The figure shows three views and two pictorial views of one solid part (mm, origin at its lowest corner). Answer the questions. A direction names the side the tool comes from. Give positions to 0.01 mm unless a question says otherwise; leave off trailing zeros. Write each loop counter-clockwise with the first axis right and the second up, starting at its lowest first coordinate (ties: lowest second). Pieces come first, ordered by that corner, then holes. Notation, with made-up numbers: (-16, 12.5) - (16, 12.5) arc R29 cw to (16, 35.5) - close; hole circle Ø5 at (-2, 79). An arc over 180 degrees is marked (long way). Use CSV: the item, a comma, the result in double quotes. Start each with the question number.
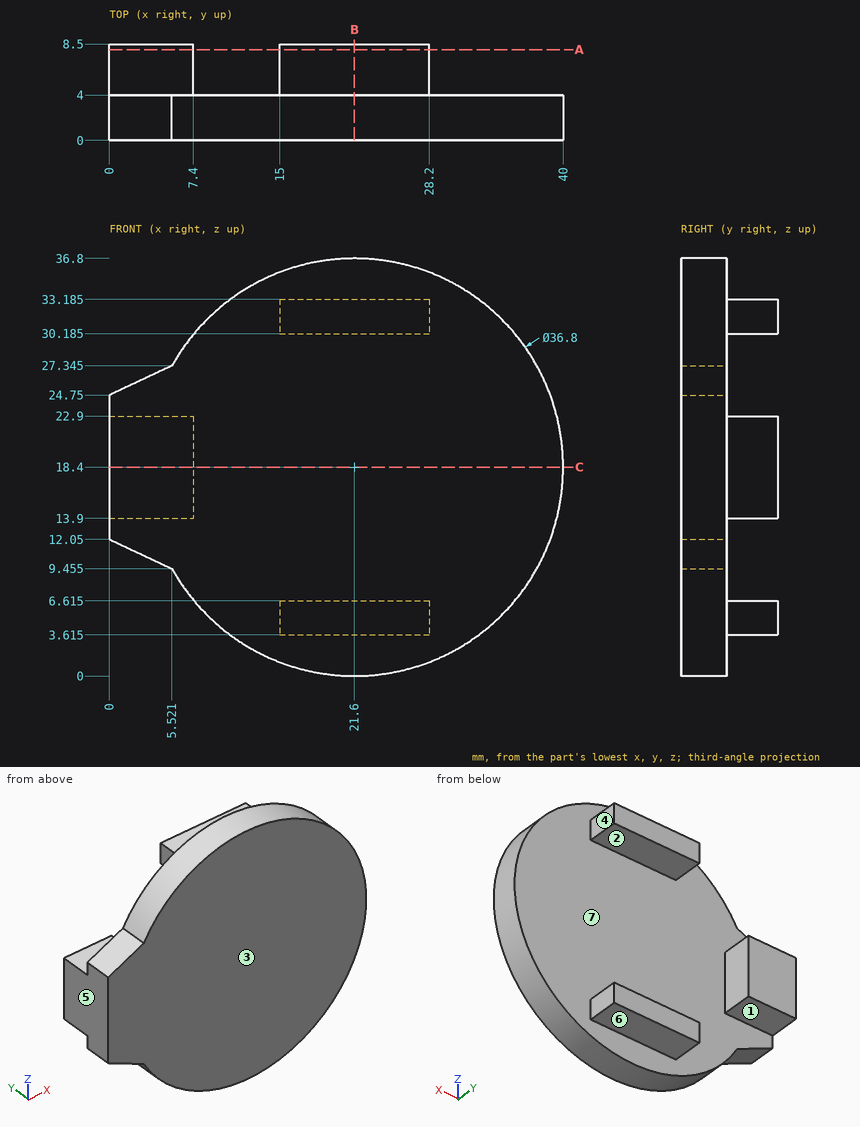
(1) Which of the six approach directions +Z, -Z, +X, -X, +Y, -Y give full straight-line access (tool end or side, diameter ignored) to the marked faces 1, 2, 3 and 4?
(2) For a pull along Z with two mould halves and no side action, classify the marked faces 5, 6 and 7 as pulls with the +Z half, pulls with the -Z half, needs draft (parallel to the pull), parting line crosses it, or undercut.
(3) The part is cut by section A-A on y = 8. Write down the section's boundary in (x, z) (1 decimal), plus the area to 3 significant figures.
(4) The part is cut by section B-B on x = 21.6. Write down the section's boundary in (y, z) (1 decimal).
(5) The part is cut by section C-C on z = 18.4. Write down the section's boundary in (x, y).
(6) Given P1, Ø2, axis at y = 3.5, z = 28.5, coming from the +X side; P2, Ø1.5, axis at x = 16.5, y = 4, coming from the +Z side; P3, Ø5, axis at x = 6, y = 4, coming from the -Z side, each flat-ended and moving along its own axis, determine where each tip first touches the part or whether it passes through.
(7) Consider probe 1 along Y at (x, z) = (37.5, 23); probe 2 along Z at (x, y) = (4.5, 6); probe 3 along X at (y, z) = (4.75, 18.5). Determine where each line is inside the solid, lowest interval first.
Reported:
1,face 1,"-Z, +X, -X, +Y"
1,face 2,"+X, -X, +Y"
1,face 3,"+Z, -Z, +X, -X, -Y"
1,face 4,"+Z, -Z, +X, +Y"
2,face 5,"needs draft"
2,face 6,"pulls with the -Z half"
2,face 7,"undercut"
3,outline,"(0, 13.9) - (7.4, 13.9) - (7.4, 22.9) - (0, 22.9) - close; (15, 3.6) - (28.2, 3.6) - (28.2, 6.6) - (15, 6.6) - close; (15, 30.2) - (28.2, 30.2) - (28.2, 33.2) - (15, 33.2) - close"
3,area,"146 mm²"
4,outline,"(0, 0) - (4, 0) - (4, 3.6) - (8.5, 3.6) - (8.5, 6.6) - (4, 6.6) - (4, 30.2) - (8.5, 30.2) - (8.5, 33.2) - (4, 33.2) - (4, 36.8) - (0, 36.8) - close"
5,outline,"(0, 0) - (40, 0) - (40, 4) - (7.4, 4) - (7.4, 8.5) - (0, 8.5) - close"
6,P1,"x = 37.59"
6,P2,"z = 36.28"
6,P3,"z = 5.48"
7,probe 1,"0 to 4"
7,probe 2,"13.9 to 22.9"
7,probe 3,"0 to 7.4"
